Geometry check sheet. Reference: the model listing, model coordinates, mm. A direction names the side the tool comes from. Coordinates: 2 decimals unless noted, no trailing zeros. Write each loop counter-clockwise with the first axis right and the second up, starting at its lowest first coordinate (ties: lowest second). Pieces come first, ordered by that corner, then holes. Notation, with made-up numbers: M 0.25,24 L 41.25,24 A19 cw 41.25,57 Z; hole C -6.5,24.5 d10. An arc over 180 degrees is marked long. Put each result on its own line as item: value. Start each with the question number.
1) Cross-section at B-B on y = 3.75. Record the cut outline in (x, z), plus the area to 3 significant figures.
2) Gauge pin test, flat ends, axial feed: pin 1 (0.6 mm diameter, centred on x = 2, y = 1, fed in from +Z); pin 2 (2 mm diameter, centred on x = 2, z = 0.5, fed in from +Y); pin 3 (0.6 mm diameter, centred on y = -3, z = -0.5, fed in from +X). Record the tip position at first contact, or that the pin passes through.
3) Scan lines: line 1 along Y through (x, z) = (2.85, 0.15); line 2 along Y through (x, z) = (2.3, 3.65); line 3 along Z through (x, y) = (0.5, -0.75). Record each from-to range of solid material in increasing order.
4) Mould release check, pull along Y, two halves, no side actions. Record for faces 5 (the flat face through (3, 0, 1.15)), 6 (the flat face through (3, -1, 1.5)): released by +Y, released by -Y, zero draft, split by the parting line, or undercut.
5) Cross-section at C-C on y = 0.5. Record the cut outline in (x, z), plus the area to 3 significant figures.
6) Set-up check for faces 1 (the flat face through (2.495, 3, 0)), 2 (the flat face through (3, 1, 1.5)), 3 (the flat face through (2.773, -3, 0)), 4 (the flat face through (3, 1.533, 0)): record each of +Z, -Z, +X, -X, +Y, -Y from which the full face is reachable in a straight line by a thin tool's end or side.
from build123d import *

# Parameters (mm, degrees)
RESSALTO_EXTRUS_O1_DEPTH = 5.25
CORTE_EXTRUS_O1_DEPTH    = 5.25
CORTE_EXTRUS_O2_DEPTH    = 5.25
FILETE1_R                = 0.2
FILETE2_R                = 0.2
ESBO_O5_W                = 0.260533882
ESBO_O5_H                = 2.040360402
RESSALTO_EXTRUS_O2_DEPTH = 2.25
ESBO_O6_W                = 0.29646959
ESBO_O6_H                = 2.02037459
RESSALTO_EXTRUS_O3_DEPTH = 2.25


with BuildPart() as part:
    # Esboço1 → Ressalto-extrusão1 (new body)
    with BuildSketch(Plane(origin=(0, 0, 0), x_dir=(0, 0, -1), z_dir=(1, 0, 0))):
        with BuildLine():
            Line((1.15, 1.533333333), (1.41, 1.533333333))
            ThreePointArc((1.41, 1.533333333), (1.47363961, 1.559693723), (1.5, 1.623333333))
            Line((1.5, 1.623333333), (1.5, 1.91))
            ThreePointArc((1.5, 1.91), (1.47363961, 1.97363961), (1.41, 2))
            Line((1.41, 2), (-1, 2))
            ThreePointArc((-1, 2), (-1.353553391, 1.853553391), (-1.5, 1.5))
            Line((-1.5, 1.5), (-1.5, 0.3))
            ThreePointArc((-1.5, 0.3), (-1.382013537, 0.239983106), (-1.299811944, 0.136225065))
            Line((-1.299811944, 0.136225065), (-4.357674279, 0.136225065))
            ThreePointArc((-4.357674279, 0.136225065), (-4.493899344, 0), (-4.357674279, -0.136225065))
            Line((-4.357674279, -0.136225065), (-1.299811944, -0.136225065))
            ThreePointArc((-1.299811944, -0.136225065), (-1.382013537, -0.239983106), (-1.5, -0.3))
            Line((-1.5, -0.3), (-1.5, -1.5))
            ThreePointArc((-1.5, -1.5), (-1.353553391, -1.853553391), (-1, -2))
            Line((-1, -2), (1.41, -2))
            ThreePointArc((1.41, -2), (1.47363961, -1.97363961), (1.5, -1.91))
            Line((1.5, -1.91), (1.5, -1.623333333))
            ThreePointArc((1.5, -1.623333333), (1.47363961, -1.559693723), (1.41, -1.533333333))
            Line((1.41, -1.533333333), (1.15, -1.533333333))
            Line((1.15, -1.533333333), (-1.15, -1.533333333))
            Line((-1.15, -1.533333333), (-1.15, 1.533333333))
            Line((-1.15, 1.533333333), (1.15, 1.533333333))
        make_face()
    extrude(amount=RESSALTO_EXTRUS_O1_DEPTH)

    # Esboço3 → Corte-extrusão1 (cut)
    with BuildSketch(Plane(origin=(0, 0.136225065, 0), x_dir=(1, 0, 0), z_dir=(0, 1, 0))):
        with BuildLine():
            Line((0.9764494, -1.514917526), (7.89407317, -1.514917526))
            ThreePointArc((7.89407317, -1.514917526), (8.3702213, -1.991065656), (7.89407317, -2.467213785))
            Line((7.89407317, -2.467213785), (0.9764494, -2.467213785))
            ThreePointArc((0.9764494, -2.467213785), (0.500301271, -1.991065656), (0.9764494, -1.514917526))
        make_face()
    extrude(amount=-CORTE_EXTRUS_O1_DEPTH, mode=Mode.SUBTRACT)

    # Esboço4 → Corte-extrusão2 (cut)
    with BuildSketch(Plane(origin=(0, 0.136225065, 0), x_dir=(1, 0, 0), z_dir=(0, 1, 0))):
        with BuildLine():
            Line((4.695795168, -2.467213785), (4.884457634, -1.937162094))
            Line((4.884457634, -1.937162094), (6.007448506, -2.098872779))
            Line((6.007448506, -2.098872779), (6.375789512, -3.266783286))
            Line((6.375789512, -3.266783286), (5.25, -3.203895797))
            ThreePointArc((5.25, -3.203895797), (5.125469424, -2.720775212), (4.695795168, -2.467213785))
        make_face()
    extrude(amount=-CORTE_EXTRUS_O2_DEPTH, mode=Mode.SUBTRACT)

    # Filete1
    filete1_edges = [part.edges().sort_by_distance(p)[0] for p in [
        (2.836122284, 0.136225065, 2.467213785),
        (3.1132247, 0.136225065, 1.514917526),
        (0.500301271, 0.136225065, 1.991065656),
    ]]
    fillet(filete1_edges, radius=FILETE1_R)

    # Filete2
    # the kernel refuses this fillet: 0.2 mm, written as the material it takes off along each edge
    with BuildSketch(Plane(origin=(5.080917151, -0.136225065, 2.467213785), x_dir=(0, 0, 1), z_dir=(-1, 0, 0))) as filete2_piece_1:
        with BuildLine():
            CenterArc((0.154048793, 0.2), FILETE2_R, 219.624198081, 50.375801919)
            Line((0, 0.07245013), (-0.003080976, 0.069899133))
            ThreePointArc((-0.003080976, 0.069899133), (-0.004, 0.036225065), (-0.004, 0))
            Line((-0.004, 0), (0, -0.004))
            Line((0, -0.004), (0.154048793, -0.004))
            Line((0.154048793, -0.004), (0.154048793, 0))
        make_face()
    extrude(amount=4.104467751, mode=Mode.SUBTRACT)
    with BuildSketch(Plane(origin=(0.9764494, -0.136225065, 1.991065656), x_dir=(0, 0, -1), z_dir=(1, 0, 0))) as filete2_piece_2:
        with BuildLine():
            CenterArc((0.630196923, 0.2), FILETE2_R, 219.624198081, 50.375801919)
            Line((0.47614813, 0.07245013), (0.473067154, 0.069899133))
            ThreePointArc((0.473067154, 0.069899133), (0.47214813, 0.036225065), (0.47214813, 0))
            Line((0.47214813, 0), (0.47614813, -0.004))
            Line((0.47614813, -0.004), (0.630196923, -0.004))
            Line((0.630196923, -0.004), (0.630196923, 0))
        make_face()
    revolve(axis=Axis((0.9764494, -0.136225065, 1.991065656), (0, 1, 0)), revolution_arc=180, mode=Mode.SUBTRACT)
    with BuildSketch(Plane(origin=(0.9764494, -0.136225065, 1.514917526), x_dir=(0, 1, 0), z_dir=(1, 0, 0))) as filete2_piece_3:
        with BuildLine():
            CenterArc((0.2, -0.154048793), FILETE2_R, 129.624198081, 50.375801919)
            Line((0, -0.154048793), (-0.004, -0.154048793))
            Line((-0.004, -0.154048793), (-0.004, 0))
            Line((-0.004, 0), (0, 0.004))
            ThreePointArc((0, 0.004), (0.036225065, 0.004), (0.069899133, 0.003080976))
            Line((0.069899133, 0.003080976), (0.07245013, 0))
        make_face()
    extrude(amount=4.658672583, mode=Mode.SUBTRACT)

    # Esboço5 → Ressalto-extrusão2 (add)
    with BuildSketch(Plane(origin=(0, 2, 0), x_dir=(1, 0, 0), z_dir=(0, 1, 0))):
        with Locations((2.625, 0.205)):
            Rectangle(ESBO_O5_W, ESBO_O5_H)
    extrude(amount=RESSALTO_EXTRUS_O2_DEPTH)

    # Esboço6 → Ressalto-extrusão3 (add)
    with BuildSketch(Plane.XZ.offset(2)):
        with Locations((2.625, -0.205)):
            Rectangle(ESBO_O6_W, ESBO_O6_H)
    extrude(amount=RESSALTO_EXTRUS_O3_DEPTH)


solid = part.part
Answer key:
1. outline: M 2.49,-1.23 L 2.76,-1.23 L 2.76,0.82 L 2.49,0.82 Z
1. area: 0.532 mm²
2. pin 1: stops at z = 1.5
2. pin 2: stops at y = 4.25
2. pin 3: stops at x = 2.77
3. line 1: y = -2 to -1.53, 1.53 to 2
3. line 2: y = -0.14 to 0.14
3. line 3: z = 1.15 to 1.5
4. face 5: undercut
4. face 6: zero draft
5. outline: M 0,1.15 L 5.25,1.15 L 5.25,1.5 L 0,1.5 Z
5. area: 1.84 mm²
6. face 1: +Z, -Z, -X, +Y
6. face 2: +Z, +X, -X, +Y
6. face 3: +Z, -Z, +X, -Y
6. face 4: -Z, +X, -X
